from build123d import *

# Parameters (mm, degrees)
BOSS_EXTRUDE1_DEPTH = 5
SKETCH11_R          = 7.25
BOSS_EXTRUDE3_DEPTH = 0.5
SKETCH12_R          = 6
BOSS_EXTRUDE4_DEPTH = 3.5
SKETCH13_R          = 1.55
CUT_EXTRUDE1_DEPTH  = 20.5
CUT_EXTRUDE2_DEPTH  = 2.6
SKETCH16_R          = 2.85
CUT_EXTRUDE3_DEPTH  = 3.02
SKETCH17_R          = 1.55
CUT_EXTRUDE4_DEPTH  = 10.02
CUT_EXTRUDE13_DEPTH = 10


with BuildPart() as part:
    # Sketch2 → Boss-Extrude1 (new body)
    with BuildSketch(Plane.XY):
        with BuildLine():
            Line((0, 11.5), (90, 11.5))
            ThreePointArc((90, 11.5), (101.5, 0), (90, -11.5))
            Line((90, -11.5), (0, -11.5))
            ThreePointArc((0, -11.5), (-11.5, 0), (0, 11.5))
        make_face()
    extrude(amount=-BOSS_EXTRUDE1_DEPTH)

    # Sketch11 → Boss-Extrude3 (add)
    with BuildSketch(Plane.XY):
        with Locations((90, 0)):
            Circle(SKETCH11_R)
    extrude(amount=BOSS_EXTRUDE3_DEPTH)

    # Sketch12 → Boss-Extrude4 (add)
    with BuildSketch(Plane.XY.offset(0.5)):
        with Locations((90, 0)):
            Circle(SKETCH12_R)
    extrude(amount=BOSS_EXTRUDE4_DEPTH)

    # Sketch13 → Cut-Extrude1 (cut)
    with BuildSketch(Plane.XY.offset(4)):
        with Locations((90, 0)):
            Circle(SKETCH13_R)
    extrude(amount=-CUT_EXTRUDE1_DEPTH, mode=Mode.SUBTRACT)

    # Sketch14 → Cut-Extrude2 (cut)
    with BuildSketch(Plane(origin=(0, 0, -5), x_dir=(-1, 0, 0), z_dir=(0, 0, -1))):
        Polygon((-93.213605432, -0.355068252), (-91.299304589, -2.960598068), (-88.085699158, -2.605529815), (-86.786394568, 0.355068252), (-88.700695411, 2.960598068), (-91.914300842, 2.605529815), align=None)
    extrude(amount=-CUT_EXTRUDE2_DEPTH, mode=Mode.SUBTRACT)

    # Sketch16 → Cut-Extrude3 (cut)
    with BuildSketch(Plane(origin=(0, 0, -5), x_dir=(-1, 0, 0), z_dir=(0, 0, -1))):
        Circle(SKETCH16_R)
    extrude(amount=-CUT_EXTRUDE3_DEPTH, mode=Mode.SUBTRACT)

    # Sketch17 → Cut-Extrude4 (cut)
    with BuildSketch(Plane.XY):
        with Locations((0, 7)):
            Circle(SKETCH17_R)
        with Locations((0, -7)):
            Circle(SKETCH17_R)
        with Locations((-7, 0)):
            Circle(SKETCH17_R)
        with Locations((7, 0)):
            Circle(SKETCH17_R)
    extrude(amount=-CUT_EXTRUDE4_DEPTH, mode=Mode.SUBTRACT)

    # Sketch18 → Cut-Extrude13 (cut)
    with BuildSketch(Plane.XY):
        Polygon((50.43728363, 8), (20.43728363, 8), (35.43728363, -8), align=None)
        with BuildLine():
            Line((30.43728363, -8), (15.43728363, 8))
            ThreePointArc((15.43728363, 8), (12.608856505, 6.828427125), (11.43728363, 4))
            Line((11.43728363, 4), (11.43728363, -4))
            ThreePointArc((11.43728363, -4), (12.608856505, -6.828427125), (15.43728363, -8))
            Line((15.43728363, -8), (30.43728363, -8))
        make_face()
        Polygon((70.43728363, -8), (55.43728363, 8), (40.43728363, -8), align=None)
        with BuildLine():
            Line((75.396348206, 8), (60.43728363, 8))
            Line((60.43728363, 8), (75.43728363, -8))
            ThreePointArc((75.43728363, -8), (78.239211349, -6.814126517), (79.396348206, -4.000209469))
            Line((79.396348206, -4.000209469), (79.396348206, 4))
            ThreePointArc((79.396348206, 4), (78.224775331, 6.828427125), (75.396348206, 8))
        make_face()
    extrude(amount=-CUT_EXTRUDE13_DEPTH, mode=Mode.SUBTRACT)


solid = part.part
Work out the finished part from the listing and answer in its coordinate system (mm). A direction names the side the tool comes from. Round coordinates to 2 decimals unless told otherwise and drop trailing zeros. Loops run counter-clockwise (first coordinate to the right, second up) from the corner with the lowest first, then second, coordinate; pieces in that order, holes last. Notation, with made-up numbers: (8.5, -15) - (61.5, -15) arc R22 ccw to (61.5, 14) - close; hole circle Ø1 at (5, 23). An arc over 180 degrees is marked (long way). Use one line per item in the form item = value. Start each with the question number.
(1) Consider line 1 (Y direction, x = 0, z = -1.05); line 2 (Y direction, x = 0, z = -2.05); line 3 (Y direction, x = 23.5, z = -3.5). Determine where each line is inside the solid, lowest interval first.
(2) Determine the mould class of faces 1 (the face through (91.25, -1.25, 4)), 2 (the face through (2.262, -1.734, -3.511)), 3 (the face through (46, -11.5, -2)) for opening direction Y: +Y half, -Y half, draft (parallel to the pull), parting line (faces both ways), or undercut.
(3) Find section C-C on x = 77.5. Determine the outline of the cut face in (y, z).
(4) Which of the six approach directions +Z, -Z, +X, -X, +Y, -Y give full straight-line access (tool end or side, diameter ignored) to faces 4 (the face through (92.3, -1.6, -3.7)), 5 (the face through (101.497, 0.253, -2.465)), 6 (the face through (12.58, -6.8, -2.46))?
(5) Find section A-A on x = 7. Determine the outline of the cut face in (y, z), and give its area (3 significant figures).
(6) Find section B-B on x = 29. Determine the outline of the cut face in (y, z).
(7) Flat-ended cylindrical pins translate along their axes: P1, Ø3, axis at x = 0, y = 7, coming from the +Z side; P2, Ø1, axis at y = -3.5, z = 2, coming from the -X side; P3, Ø2.5, axis at y = -1, z = -1.5, coming from the -X side; P4, Ø3, axis at y = -5, z = -4, coming from the +X side. Find the tip coordinate at first contact, or state that the pin passes through.
Answer list:
q1.line_1 = -11.5 to -8.55, -5.45 to 5.45, 8.55 to 11.5
q1.line_2 = -11.5 to -8.55, -5.45 to -2.85, 2.85 to 5.45, 8.55 to 11.5
q1.line_3 = -11.5 to -8, -0.6 to 4.73, 8 to 11.5
q2.face_1 = draft
q2.face_2 = undercut
q2.face_3 = -Y half
q3.outline = (-11.5, -5) - (-7.4, -5) - (-7.4, 0) - (-11.5, 0) - close; (7.4, -5) - (11.5, -5) - (11.5, 0) - (7.4, 0) - close
q4.face_4 = -Z
q4.face_5 = +Z, -Z, +X
q4.face_6 = +Z, -Z
q5.outline = (-11.5, -5) - (-1.55, -5) - (-1.55, 0) - (-11.5, 0) - close; (1.55, -5) - (11.5, -5) - (11.5, 0) - (1.55, 0) - close
q5.area = 99.5 mm^2
q6.outline = (-11.5, -5) - (-8, -5) - (-8, 0) - (-11.5, 0) - close; (-6.47, -5) - (-1.13, -5) - (-1.13, 0) - (-6.47, 0) - close; (8, -5) - (11.5, -5) - (11.5, 0) - (8, 0) - close
q7.P1 = through
q7.P2 = 84.8
q7.P3 = -11.5
q7.P4 = 100.95
